Part print with two shaded views. Sizes in mm from the minimum x, y, z corner. A direction names the side the tool comes from. Coordinates: 2 decimals unless noted, no trailing zeros. Write each loop counter-clockwise with the first axis right and the second up, starting at its lowest first coordinate (ties: lowest second). Pieces come first, ordered by that corner, then holes.
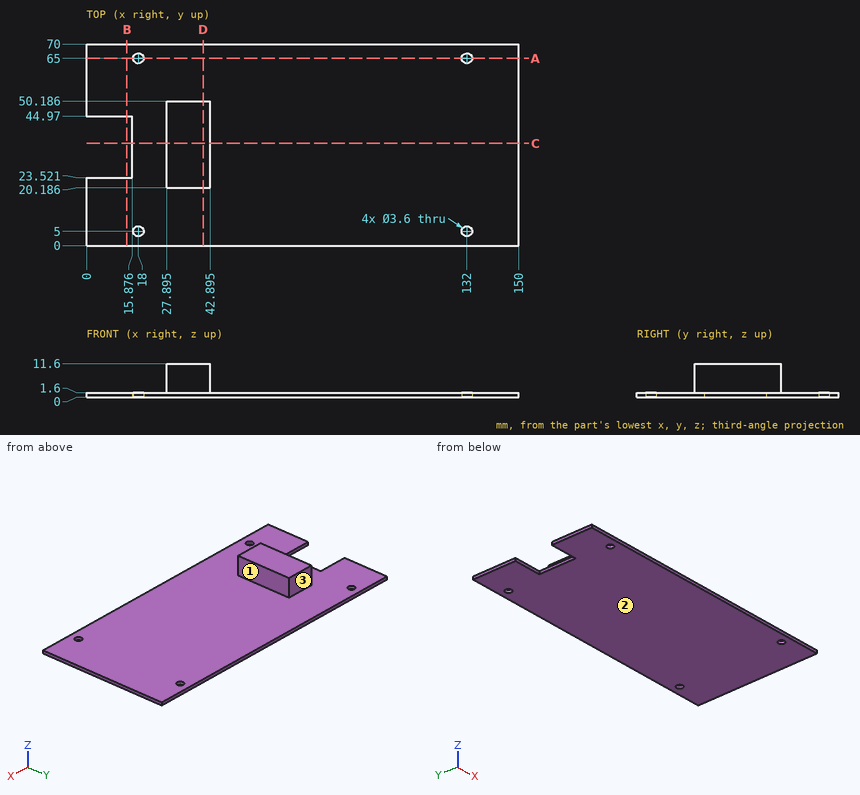
(1) Slice it at A-A, the plane y = 65. List the corners of the cut face in (x, z).
(2) Slice it at D-D, the plane x = 40.5. List the corners of the cut face in (y, z), and give its area (3 significant figures).
(3) Slice it at C-C, the plane y = 35.5. List the corners of the cut face in (x, z) (1 decimal).
(4) 3-axis set-ups, long thin cutter, end or side, ignore diameter. For the marked faces 1, 2 and 3: which of +Z, -Z, +X, -X, +Y, -Y reach the whole face in a straight line?
(5) Probe L1, parallel to Y at x = 18, z = 0.95; L2, parallel to X at y = 65, z = 1.25; L3, parallel to X at y = 24, z = 2.5 (1 decimal). List the from-to ranges inside material, lowest first.
(6) Slice it at B-B, the plane x = 14. List the corners of the cut face in (y, z).
(7) Flat gauge pins, fed straight in: P1, Ø3, axis at y = 36, z = 6, coming from the +X side (1 decimal); P2, Ø3, axis at x = 78.5, y = 55, coming from the +Z side; P3, Ø1.5, axis at x = 39, z = 7, coming from the +Y side; P4, Ø3, axis at x = 132, y = 5, coming from the -Z side. Where does each tip first touch, or does it go through?
Results:
1. outline: (0, 0) - (16.2, 0) - (16.2, 1.6) - (0, 1.6) - close; (19.8, 0) - (130.2, 0) - (130.2, 1.6) - (19.8, 1.6) - close; (133.8, 0) - (150, 0) - (150, 1.6) - (133.8, 1.6) - close
2. outline: (0, 0) - (70, 0) - (70, 1.6) - (50.19, 1.6) - (50.19, 11.6) - (20.19, 11.6) - (20.19, 1.6) - (0, 1.6) - close
2. area: 412 mm2
3. outline: (15.9, 0) - (150, 0) - (150, 1.6) - (42.9, 1.6) - (42.9, 11.6) - (27.9, 11.6) - (27.9, 1.6) - (15.9, 1.6) - close
4. face 1: +Z, +X, +Y, -Y
4. face 2: -Z, +X, -X, +Y, -Y
4. face 3: +Z, +X, -X, +Y
5. L1: y = 0 to 3.2, 6.8 to 63.2, 66.8 to 70
5. L2: x = 0 to 16.2, 19.8 to 130.2, 133.8 to 150
5. L3: x = 27.9 to 42.9
6. outline: (0, 0) - (23.52, 0) - (23.52, 1.6) - (0, 1.6) - close; (44.97, 0) - (70, 0) - (70, 1.6) - (44.97, 1.6) - close
7. P1: stops at x = 42.9
7. P2: stops at z = 1.6
7. P3: stops at y = 50.19
7. P4: passes through
